Source: CAD feature listing. Evaluate the final solid. Frame: model axes, mm. A direction names the side the tool comes from. Round coordinates to 2 decimals unless told otherwise and drop trailing zeros. Order: outer loops, then holes, each group sorted by start corner. A loop starts at its lowest first (then second) coordinate and runs counter-clockwise, first axis right, second up. Notation, with made-up numbers: (0, 64.5) -> (22, 64.5) arc R18 cw to (22, 84.5) -> close; hole circle Ø10 at (85, 82.25). An arc over 180 degrees is marked (long way). Use a Markdown table: item, result. Add a question column.
```python
from build123d import *

# Parameters (mm, degrees)
SKETCH1_W               = 40
SKETCH1_H               = 20
BOSS_EXTRUDE1_DEPTH     = 8
SKETCH2_W               = 40
SKETCH2_H               = 8
BOSS_EXTRUDE2_DEPTH     = 16
SKETCH4_R               = 3.15
CUT_EXTRUDE1_DEPTH      = 38.094473982
SKETCH5_R               = 1.6
CUT_EXTRUDE2_DEPTH      = 8
SKETCH6_R               = 1.6
CUT_EXTRUDE3_DEPTH      = 8
CUT_EXTRUDE4_DEPTH      = 33.802438934
CUT_EXTRUDE4_DEPTH_BACK = 1.6
SKETCH9_R               = 3
CUT_EXTRUDE5_DEPTH      = 4
SKETCH10_R              = 3
CUT_EXTRUDE6_DEPTH      = 4
CUT_EXTRUDE7_DEPTH      = 4
FILLET1_R               = 10


with BuildPart() as part:
    # Sketch1 → Boss-Extrude1 (new body)
    with BuildSketch(Plane.XY):
        Rectangle(SKETCH1_W, SKETCH1_H)
    extrude(amount=BOSS_EXTRUDE1_DEPTH)

    # Sketch2 → Boss-Extrude2 (add)
    with BuildSketch(Plane.XY.offset(8)):
        with Locations((0, 6)):
            Rectangle(SKETCH2_W, SKETCH2_H)
    extrude(amount=BOSS_EXTRUDE2_DEPTH)

    # Sketch4 → Cut-Extrude1 (cut, through all)
    with BuildSketch(Plane(origin=(0, 10, 0), x_dir=(1, 0, 0), z_dir=(0, 1, 0))):
        with Locations(Location((0, -14, 0), (0, 0, 270))):
            Circle(SKETCH4_R)
    extrude(amount=-CUT_EXTRUDE1_DEPTH, mode=Mode.SUBTRACT)

    # Sketch5 → Cut-Extrude2 (cut)
    with BuildSketch(Plane(origin=(0, 0, 0), x_dir=(-1, 0, 0), z_dir=(0, 0, -1))):
        with Locations((-15, -2.5)):
            Circle(SKETCH5_R)
    extrude(amount=-CUT_EXTRUDE2_DEPTH, mode=Mode.SUBTRACT)

    # Sketch6 → Cut-Extrude3 (cut)
    with BuildSketch(Plane(origin=(0, 0, 0), x_dir=(-1, 0, 0), z_dir=(0, 0, -1))):
        with Locations((15, -2.5)):
            Circle(SKETCH6_R)
    extrude(amount=-CUT_EXTRUDE3_DEPTH, mode=Mode.SUBTRACT)

    # Sketch7 → Cut-Extrude4 (cut, two sides: drawn at the far end of the back side and taken through both)
    with BuildSketch(Plane(origin=(0, 0, 0), x_dir=(-1, 0, 0), z_dir=(0, 0, -1)).offset(-CUT_EXTRUDE4_DEPTH_BACK)):
        Polygon((-11, -93.783466983), (-11, -10), (-11, 2.5), (-7.5, 2.5), (-7.5, 6.5), (7.5, 6.5), (7.5, 2.5), (11, 2.5), (11, -10), (11, -93.783466983), (11, -261.350400948), (-11, -261.350400948), align=None)
    extrude(amount=CUT_EXTRUDE4_DEPTH + CUT_EXTRUDE4_DEPTH_BACK, mode=Mode.SUBTRACT)

    # Sketch9 → Cut-Extrude5 (cut)
    with BuildSketch(Plane.XY.offset(8)):
        with Locations((-15, -2.5)):
            Circle(SKETCH9_R)
    extrude(amount=-CUT_EXTRUDE5_DEPTH, mode=Mode.SUBTRACT)

    # Sketch10 → Cut-Extrude6 (cut)
    with BuildSketch(Plane.XY.offset(8)):
        with Locations((15, -2.5)):
            Circle(SKETCH10_R)
    extrude(amount=-CUT_EXTRUDE6_DEPTH, mode=Mode.SUBTRACT)

    # Sketch11 → Cut-Extrude7 (cut)
    with BuildSketch(Plane.XZ.offset(-2)):
        Polygon((6.062177826, 14), (3.031088913, 19.25), (-3.031088913, 19.25), (-6.062177826, 14), (-3.031088913, 8.75), (3.031088913, 8.75), align=None)
    extrude(amount=-CUT_EXTRUDE7_DEPTH, mode=Mode.SUBTRACT)

    # Fillet1
    fillet1_edges = [part.edges().sort_by_distance(p)[0] for p in [
        (-20, 6, 24),
        (20, 6, 24),
    ]]
    fillet(fillet1_edges, radius=FILLET1_R)


solid = part.part
```
1) Draft query along Z for faces 6 (the flat face through (0, 4, 8.75)), 7 (the flat face through (-20, 2, 5)), 8 (the flat face through (0, -4, 8)). Return one class per face: pulls with the +Z half, pulls with the -Z half, needs draft (parallel to the pull), parting line crosses it, or undercut.
2) Line query: probe 1 along Y at (x, z) = (-15, 2.8); probe 2 along Z at (x, y) = (-2.5, 3.5); probe 3 along Z at (x, y) = (-7.5, -4.5). Output: solid intervals per line, ascending. Write a range as from..to.
3) Reachability of faces 1 (the flat face through (0, 7, 0)), 2 (the flat face through (16, -4, 4)), 3 (the flat face through (-0.28, 2, 19.44)), 4 (the flat face through (-9, 2.5, 1)), 5 (the flat face through (3, 6, 16)) from +Z, -Z, +X, -X, +Y, -Y: full face, straight path, thin tool, end or side. Return the list, or none.
4) Section B-B on x = 0. Output: boundary loops of the cut face in (y, z).
5) First-contact query: pin 1 Ø2 at (x, z) = (10, 17) entering from -Y; pin 2 Ø1.5 at (x, y) = (-2, 3.5) entering from -Z; pin 3 Ø1.5 at (x, y) = (-3.5, -1) entering from +Z. Flat tips, straight axial feed; report the tip coordinate or a pass-through.
6) Section C-C on y = -2.5. Output: boundary loops of the cut face in (x, z), then the cut area to 3 significant figures.
7) Section D-D on z = 6.75. Output: boundary loops of the cut face in (x, y).
8) Section A-A on y = 4.5. Output: boundary loops of the cut face in (x, z), then the cut area to 3 significant figures.
Conclusion:
| question | item | result |
|---|---|---|
| 1 | face 6 | undercut |
| 1 | face 7 | needs draft |
| 1 | face 8 | pulls with the +Z half |
| 2 | probe 1 | y = -10..-4.1, -0.9..10 |
| 2 | probe 2 | z = 1.6..8.75, 19.25..24 |
| 2 | probe 3 | z = 1.6..8 |
| 3 | face 1 | -Z, +X, -X, +Y, -Y |
| 3 | face 2 | +Z |
| 3 | face 3 | +Z, +X, -X, -Y |
| 3 | face 4 | -Z, -Y |
| 3 | face 5 | -Y |
| 4 | outline | (-10, 1.6) -> (6.5, 1.6) -> (6.5, 0) -> (10, 0) -> (10, 10.85) -> (6, 10.85) -> (6, 8.75) -> (2, 8.75) -> (2, 8) -> (-10, 8) -> close; (2, 19.25) -> (6, 19.25) -> (6, 17.15) -> (10, 17.15) -> (10, 24) -> (2, 24) -> close |
| 5 | pin 1 | stops at y = 2 |
| 5 | pin 2 | stops at z = 1.6 |
| 5 | pin 3 | stops at z = 8 |
| 6 | outline | (-20, 0) -> (-16.6, 0) -> (-16.6, 4) -> (-18, 4) -> (-18, 8) -> (-20, 8) -> close; (-13.4, 0) -> (-11, 0) -> (-11, 1.6) -> (11, 1.6) -> (11, 0) -> (13.4, 0) -> (13.4, 4) -> (12, 4) -> (12, 8) -> (-12, 8) -> (-12, 4) -> (-13.4, 4) -> close; (16.6, 0) -> (20, 0) -> (20, 8) -> (18, 8) -> (18, 4) -> (16.6, 4) -> close |
| 6 | area | 211 mm^2 |
| 7 | outline | (-20, -10) -> (20, -10) -> (20, 10) -> (-20, 10) -> close; hole circle Ø6 at (-15, -2.5); hole circle Ø6 at (15, -2.5) |
| 8 | outline | (-20, 0) -> (-7.5, 0) -> (-7.5, 1.6) -> (7.5, 1.6) -> (7.5, 0) -> (20, 0) -> (20, 14) arc R10 ccw to (10, 24) -> (-10, 24) arc R10 ccw to (-20, 14) -> close; hole (-6.06, 14) -> (-3.03, 8.75) -> (3.03, 8.75) -> (6.06, 14) -> (3.03, 19.25) -> (-3.03, 19.25) -> close |
| 8 | area | 798 mm^2 |
